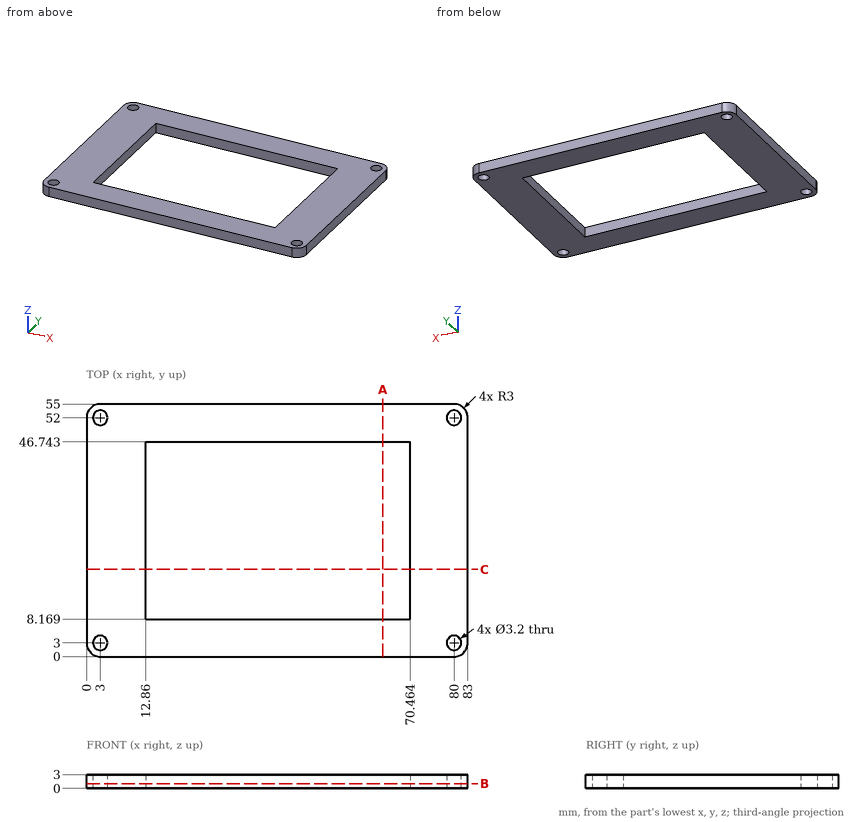
Study the drawing (mm; zero at the part's minimum x, y, z) and answer. Coordinates: 2 decimals unless noted, no trailing zeros. Loops run counter-clockwise (first coordinate to the right, second up) from the corner with the lowest first, then second, coordinate; pieces in that order, holes last. Notation, with made-up numbers: (27, -13) -> (51, -13) arc R19 ccw to (51, -4) -> close; hole circle Ø10 at (74, 13.5). An arc over 180 degrees is marked (long way). Write item = value, one per line. Start each with the question number.
1) The part is cut by section C-C, the plane y = 19. Determine the outline of the cut face in (x, z) (1 decimal).
2) The part is cut by section B-B, the plane z = 1.05. Determine the outline of the cut face in (x, y) (1 decimal), plus the area to 3 significant figures.
3) The part is cut by section A-A, the plane x = 64.5. Determine the outline of the cut face in (y, z).
4) Find the intervals of material crossed by L1, parallel to Y at x = 3, z = 2.1; L2, parallel to Y at x = 67, z = 0.5; L3, parallel to X at y = 42.5, z = 2.05 (1 decimal), in increasing order. Write a range as from..to.
Result:
q1.outline = (0, 0) -> (12.9, 0) -> (12.9, 3) -> (0, 3) -> close; (70.5, 0) -> (83, 0) -> (83, 3) -> (70.5, 3) -> close
q2.outline = (0, 3) arc R3 ccw to (3, 0) -> (80, 0) arc R3 ccw to (83, 3) -> (83, 52) arc R3 ccw to (80, 55) -> (3, 55) arc R3 ccw to (0, 52) -> close; hole circle Ø3.2 at (3, 3); hole circle Ø3.2 at (3, 52); hole (12.9, 8.2) -> (70.5, 8.2) -> (70.5, 46.7) -> (12.9, 46.7) -> close; hole circle Ø3.2 at (80, 3); hole circle Ø3.2 at (80, 52)
q2.area = 2,300 mm²
q3.outline = (0, 0) -> (8.17, 0) -> (8.17, 3) -> (0, 3) -> close; (46.74, 0) -> (55, 0) -> (55, 3) -> (46.74, 3) -> close
q4.L1 = 0..1.4, 4.6..50.4, 53.6..55
q4.L2 = 0..8.17, 46.74..55
q4.L3 = 0..12.9, 70.5..83
